Work out the finished part from the listing and answer in its coordinate system (mm). Face numbers are marked on the shaded views. A direction names the side the tool comes from. Give positions to 0.01 mm unless a question says otherwise; leave off trailing zeros. Loops run counter-clockwise (first coordinate to the right, second up) from the corner with the lowest first, then second, coordinate; pieces in that order, holes last. Notation, with made-up numbers: (21, 38.25) -> (69, 38.25) arc R31 cw to (69, 68.25) -> close; hole circle Ø9 at (16.5, 4). An arc over 180 degrees is marked (long way). Answer as CSV lines item,"result". Start each with the question number.
1. Determine the mould class of the marked faces 3, 4, 5 and 6 for opening direction X: +X half, -X half, draft (parallel to the pull), parting line (faces both ways), or undercut.
2. Find the intervals of material crossed by line 1 along Y through (x, z) = (-95, 6); line 2 along X through (y, z) = (7, -17) (3 decimals), in increasing order.
3. Find section B-B, the plane z = -3. Give the vertices of the cut face in (x, y) (3 decimals), and give its area (3 significant figures).
4. Find section C-C, the plane x = -14.5. Give the vertices of the cut face in (y, z).
5. A tool of negligible diameter and unlimited length cuts with its end or side. For the marked faces 1 and 2, from which of +Z, -Z, +X, -X, +Y, -Y can it reach the whole face along a straight path? Write none if from no direction.
6. Flat-ended cylindrical pins translate along their axes: pin 1 Ø2 at (x, y) = (95.25, -7.62) entering from +Z; pin 2 Ø1.9 at (x, z) = (-125.5, -19.5) entering from +Y; pin 3 Ø8 at (x, z) = (114, -37.5) entering from +Y; pin 4 Ø3 at (x, z) = (-7, 0.5) entering from -Y. Find the tip coordinate at first contact, or state that the pin passes through.
7. Find section A-A, the plane z = 8. Give the vertices of the cut face in (x, y) (3 decimals).
from build123d import *

# Parameters (mm, degrees)
SKETCH1_W           = 260.35
SKETCH1_H           = 38.1
SKETCH1_R           = 3.175
SKETCH1_R_2         = 1.85
BOSS_EXTRUDE1_DEPTH = 12.7
SKETCH2_W           = 6.35
SKETCH2_H           = 31.75
BOSS_EXTRUDE2_DEPTH = 50.8
CUT_EXTRUDE1_DEPTH  = 50.8
BOSS_EXTRUDE3_DEPTH = 5.08
CHAMFER1_SIZE       = 0.5


# Read off the part's stored shape, not the designer's step: Mirror1
with BuildPart() as part:
    # Sketch1 → Boss-Extrude1 (new body)
    with BuildSketch(Plane.XY):
        Rectangle(SKETCH1_W, SKETCH1_H)
        with Locations((-117.475, 0)):
            Circle(SKETCH1_R, mode=Mode.SUBTRACT)
        with Locations(Location((117.475, 0, 0), (0, 0, 180))):
            Circle(SKETCH1_R, mode=Mode.SUBTRACT)
        with Locations((-95.25, 12.7)):
            Circle(SKETCH1_R_2, mode=Mode.SUBTRACT)
        with Locations(Location((-95.25, -7.62, 0), (0, 0, 180))):
            Circle(SKETCH1_R_2, mode=Mode.SUBTRACT)
        with Locations((95.25, -7.62)):
            Circle(SKETCH1_R_2, mode=Mode.SUBTRACT)
        with Locations(Location((95.25, 12.7, 0), (0, 0, 180))):
            Circle(SKETCH1_R_2, mode=Mode.SUBTRACT)
    extrude(amount=BOSS_EXTRUDE1_DEPTH)

    # Sketch2 → Boss-Extrude2 (add)
    with BuildSketch(Plane(origin=(0, 0, 0), x_dir=(-1, 0, 0), z_dir=(0, 0, -1))):
        with Locations((-127, -3.175)):
            Rectangle(SKETCH2_W, SKETCH2_H)
    extrude(amount=BOSS_EXTRUDE2_DEPTH)

    # Sketch3 → Cut-Extrude1 (cut)
    with BuildSketch(Plane.ZY.offset(-123.825)):
        with BuildLine():
            Line((-38.1, 6.35), (-12.7, 6.35))
            ThreePointArc((-12.7, 6.35), (-9.525, 3.175), (-12.7, 0))
            Line((-12.7, 0), (-38.1, 0))
            ThreePointArc((-38.1, 0), (-41.275, 3.175), (-38.1, 6.35))
        make_face()
        with BuildLine():
            Line((-38.1, -8.89), (-12.7, -8.89))
            ThreePointArc((-12.7, -8.89), (-9.525, -12.065), (-12.7, -15.24))
            Line((-12.7, -15.24), (-38.1, -15.24))
            ThreePointArc((-38.1, -15.24), (-41.275, -12.065), (-38.1, -8.89))
        make_face()
    extrude(amount=-CUT_EXTRUDE1_DEPTH, mode=Mode.SUBTRACT)

    # Sketch4 → Boss-Extrude3 (add)
    with BuildSketch(Plane(origin=(0, -19.05, 0), x_dir=(-1, 0, 0), z_dir=(0, -1, 0))):
        Polygon((-123.825, 50.8), (-97.1, 0), (-97.1, -12.7), (-130.175, -12.7), (-130.175, 50.8), align=None)
    extrude(amount=BOSS_EXTRUDE3_DEPTH)

    # Mirror1: part across plane


with BuildPart() as part_1:
    add(part.part)
    add(part.part.mirror(Plane(origin=(0, 0, 0), x_dir=(0, 0, 1), z_dir=(1, 0, 0))))

    # Chamfer1
    chamfer1_edges = [part_1.edges().sort_by_distance(p)[0] for p in [
        (-120.65, 0, 12.7),
        (-130.175, -2.54, 12.7),
        (120.65, 0, 12.7),
        (0, -19.05, 12.7),
        (-113.6375, -24.13, 12.7),
        (-97.1, -21.59, 12.7),
        (-93.4, -7.62, 12.7),
        (-97.1, 12.7, 12.7),
        (93.4, -7.62, 12.7),
        (97.1, 12.7, 12.7),
        (130.175, -2.54, 12.7),
        (0, 19.05, 12.7),
        (97.1, -21.59, 12.7),
        (113.6375, -24.13, 12.7),
    ]]
    chamfer(chamfer1_edges, length=CHAMFER1_SIZE)


solid = part_1.part
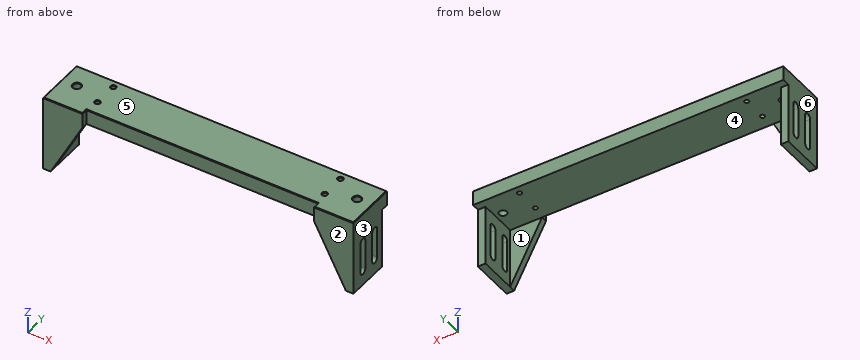
Resolved:
1,face 3,"+X half"
1,face 4,"undercut"
1,face 5,"draft"
1,face 6,"-X half"
2,line 1,"y = -19.05 to -9.45, -5.79 to 10.87, 14.53 to 19.05"
2,line 2,"x = -130.175 to -123.825, 123.825 to 130.175"
3,outline,"(-130.175, -24.13) -> (-98.678, -24.13) -> (-98.678, -19.05) -> (-123.825, -19.05) -> (-123.825, 12.7) -> (-130.175, 12.7) -> close; (98.678, -24.13) -> (130.175, -24.13) -> (130.175, 12.7) -> (123.825, 12.7) -> (123.825, -19.05) -> (98.678, -19.05) -> close"
3,area,"723 mm^2"
4,outline,"(-19.05, 0) -> (19.05, 0) -> (19.05, 12.2) -> (18.55, 12.7) -> (-18.55, 12.7) -> (-19.05, 12.2) -> close"
5,face 1,"-Z, +Y"
5,face 2,"+Z, -Z, +X, -X, -Y"
6,pin 1,"passes through"
6,pin 2,"stops at y = 12.7"
6,pin 3,"stops at y = -19.05"
6,pin 4,"stops at y = -19.05"
7,outline,"(-130.175, -24.13) -> (-97.1, -24.13) -> (-97.1, -19.05) -> (97.1, -19.05) -> (97.1, -24.13) -> (130.175, -24.13) -> (130.175, 19.05) -> (-130.175, 19.05) -> close; hole circle Ø6.35 at (-117.475, 0); hole circle Ø3.7 at (-95.25, -7.62); hole circle Ø3.7 at (-95.25, 12.7); hole circle Ø3.7 at (95.25, -7.62); hole circle Ø3.7 at (95.25, 12.7); hole circle Ø6.35 at (117.475, 0)"
